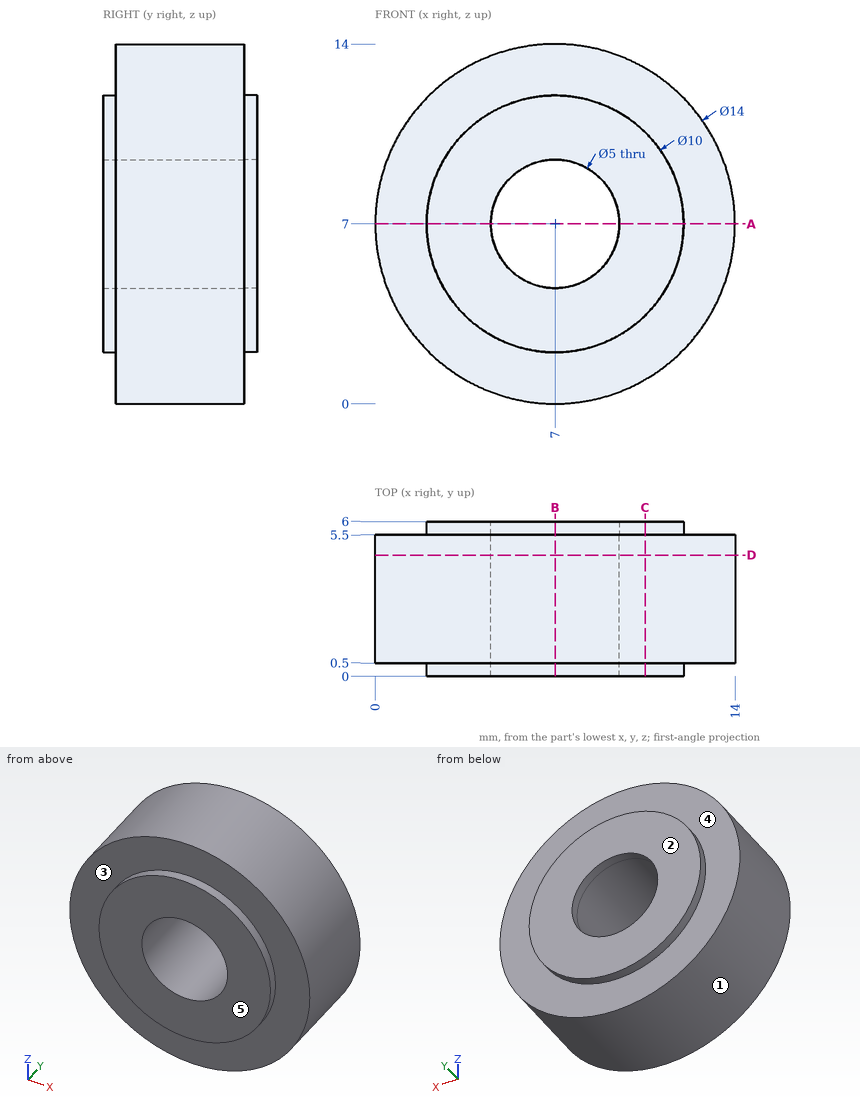
Verification items for this drawing (mm, ordinates from the low corner). A direction names the side the tool comes from. Give positions to 0.01 mm unless a question says otherwise; leave off trailing zeros. Write each loop counter-clockwise with the first axis right and the second up, starting at its lowest first coordinate (ties: lowest second). Pieces come first, ordered by that corner, then holes.
1) Access from +Z, -Z, +X, -X, +Y, -Y to the whole of each face (thin tool, end or side, straight path). Record for the marked faces 3, 4 and 5.
2) Section check B-B, the plane x = 7. Record the boundary of the cut face in (y, z), and give its area (3 significant figures).
3) Section check D-D, the plane y = 4.7. Record the boundary of the cut face in (x, z), and give its area (3 significant figures).
4) Release check for a two-part mould opening along X. For the marked faces 1 and 2 record: pulls with the +X half, pulls with the -X half, needs draft (parallel to the pull), parting line crosses it, or undercut.
5) Section check C-C, the plane x = 10.5. Record the boundary of the cut face in (y, z), and give its area (3 significant figures).
6) Section check A-A, the plane z = 7. Record the boundary of the cut face in (x, y), and give its area (3 significant figures).
7) Material ranges on L1, parallel to Z at x = 7, y = 1.65; L2, parallel to Z at x = 7, y = 5.8; L3, parallel to Y at x = 4.75, z = 12.5, recorded low to high.
8) Gauge pin test, flat ends, axial feed: pin 1 (1 mm diameter, centred on y = 3, z = 10.5, fed in from -X); pin 2 (2 mm diameter, centred on x = 10, y = 2.5, fed in from -Z); pin 3 (3 mm diameter, centred on x = 4.5, y = 1, fed in from +Z). Record the tip position at first contact, or that the pin passes through.
Computed:
1. face 3: -Y
1. face 4: +Y
1. face 5: +Z, -Z, +X, -X, -Y
2. outline: (0, 2) - (0.5, 2) - (0.5, 0) - (5.5, 0) - (5.5, 2) - (6, 2) - (6, 4.5) - (0, 4.5) - close; (0, 9.5) - (6, 9.5) - (6, 12) - (5.5, 12) - (5.5, 14) - (0.5, 14) - (0.5, 12) - (0, 12) - close
2. area: 50.0 mm2
3. outline: circle Ø14 at (7, 7); hole circle Ø5 at (7, 7)
3. area: 134 mm2
4. face 1: parting line crosses it
4. face 2: needs draft
5. outline: (0, 3.43) - (0.5, 3.43) - (0.5, 0.94) - (5.5, 0.94) - (5.5, 3.43) - (6, 3.43) - (6, 10.57) - (5.5, 10.57) - (5.5, 13.06) - (0.5, 13.06) - (0.5, 10.57) - (0, 10.57) - close
5. area: 67.8 mm2
6. outline: (0, 0.5) - (2, 0.5) - (2, 0) - (4.5, 0) - (4.5, 6) - (2, 6) - (2, 5.5) - (0, 5.5) - close; (9.5, 0) - (12, 0) - (12, 0.5) - (14, 0.5) - (14, 5.5) - (12, 5.5) - (12, 6) - (9.5, 6) - close
6. area: 50.0 mm2
7. L1: z = 0 to 4.5, 9.5 to 14
7. L2: z = 2 to 4.5, 9.5 to 12
7. L3: y = 0.5 to 5.5
8. pin 1: stops at x = 0.68
8. pin 2: stops at z = 0.29
8. pin 3: stops at z = 13.93
